from build123d import *

# Parameters (mm, degrees)
F0_W     = 50.8
F0_H     = 50.8
F1_DEPTH = 50.8
F3_R     = 25.39999
F2_R     = 23.495
F4_DEPTH = 45.72


# Not quite as in the source:
# - a fillet or chamfer is up to 0.001 mm smaller than in the source, because OpenCascade refuses the exact size


with BuildPart() as f1:
    # F0 (on Top) → F1 (new body)
    with BuildSketch(Plane.XY):
        with Locations((-25.4, 25.4)):
            Rectangle(F0_W, F0_H)
    extrude(amount=F1_DEPTH)

    # F3 (radius 25.4 in the source; OpenCascade refuses exactly that, so slightly less here)
    f3_edges = [f1.edges().sort_by_distance(p)[0] for p in [
        (0, 25.4, 50.8),
        (-50.8, 25.4, 50.8),
    ]]
    fillet(f3_edges, radius=F3_R)

    # F2 (on face) → F4 (cut)
    with BuildSketch(Plane(origin=(0, 50.8, 0), x_dir=(-1, 0, 0), z_dir=(0, 1, 0))):
        with Locations((25.4, 24.765)):
            Circle(F2_R)
    extrude(amount=-F4_DEPTH, mode=Mode.SUBTRACT)


solid = f1.part
Input: part model. Units: mm. Frame: model coordinates. A direction names the side the tool comes from. Give positions to 0.01 mm unless a question says otherwise; leave off trailing zeros. Order: outer loops, then holes, each group sorted by start corner. A loop starts at its lowest first (then second) coordinate and runs counter-clockwise, first axis right, second up. Notation, with made-up numbers: (38, 54) - (55, 54) arc R15 cw to (55, 58) - close; hole circle Ø4 at (16, 77.25). An arc over 180 degrees is marked (long way). Write each question's results on one line, items separated by ' | '.
Item 1: Contact query for flat-ended pins moving along their axis: pin 1 Ø1.5 at (x, y) = (-15.5, 15) entering from +Z; pin 2 Ø2 at (x, z) = (-12.5, 8) entering from -Y; pin 3 Ø1.5 at (y, z) = (14, 27) entering from +X; pin 4 Ø12 at (x, z) = (-12.5, 20) entering from +Y. Output: stop coordinate, or through.
A:
pin 1: stops at z = 49.09 | pin 2: stops at y = 0 | pin 3: stops at x = -0.01 | pin 4: stops at y = 5.08
Item 2: Access query for faces 1 (the flat face through (-26, 0, 25)), 2 (the cylindrical face through (-20.31, 28.26, 1.83)). Directions: +Z, -Z, +X, -X, +Y, -Y. A direction counts if a zero-diameter tool reaches every point of the face in a straight line with its end or side. Return the directions, or none.
A:
face 1: +Z, -Z, +X, -X, -Y | face 2: +Y
Item 3: Draft query along Z for faces 3 (the flat face through (0, 25, 13)), 4 (the flat face through (-26, 26, 0)), 5 (the flat face through (-25, 5.08, 25)). Return one class per face: released by +Z, released by -Z, zero draft, split by the parting line, or undercut.
A:
face 3: zero draft | face 4: released by -Z | face 5: undercut
Item 4: Section C-C (z = 34.5). Return loops of the section in (x, y).
A:
outline: (-49.11, 0) - (-1.69, 0) - (-1.69, 50.8) - (-4.02, 50.8) - (-4.02, 5.08) - (-46.78, 5.08) - (-46.78, 50.8) - (-49.11, 50.8) - close
Item 5: Section B-B (x = -41.5). Return loops of the section in (y, z), and give its area (3 significant figures).
A:
outline: (0, 0) - (50.8, 0) - (50.8, 7.65) - (5.08, 7.65) - (5.08, 41.88) - (50.8, 41.88) - (50.8, 45.05) - (0, 45.05) - close | area: 724 mm^2
Item 6: Material intervals for line 1 along Z through (x, y) = (-25, 23.5); line 2 along X through (y, z) = (26, 24); line 3 along Y through (x, z) = (-45, 22.5), sorted ascending.
A:
line 1: z = 0 to 1.27, 48.26 to 50.8 | line 2: x = -50.8 to -48.88, -1.92 to 0 | line 3: y = 0 to 5.08
